```python
from build123d import *

# Parameters (mm, degrees)
SKETCH_R  = 0.7
PAD_DEPTH = 0.25


with BuildPart() as part:
    # Sketch → Pad (new body, symmetric)
    with BuildSketch(Plane.XZ):
        with BuildLine():
            Line((-1.2, 7), (-1.2, 0))
            Line((-1.2, 0), (-0.45, 0))
            Line((-0.45, 0), (-0.45, -2.55))
            ThreePointArc((-0.45, -2.55), (0, -3), (0.45, -2.55))
            Line((0.45, 0), (0.45, -2.55))
            Line((0.45, 0), (1.2, 0))
            Line((1.2, 0), (1.2, 7))
            Line((1.2, 7), (0.7, 7))
            Line((0.7, 7), (0.7, 5.775))
            ThreePointArc((-0.7, 5.775), (0, 5.075), (0.7, 5.775))
            Line((-0.7, 5.775), (-0.7, 7))
            Line((-0.7, 7), (-1.2, 7))
        make_face()
        with Locations((0, 2.3331)):
            Circle(SKETCH_R, mode=Mode.SUBTRACT)
    extrude(amount=PAD_DEPTH, both=True)


solid = part.part
```
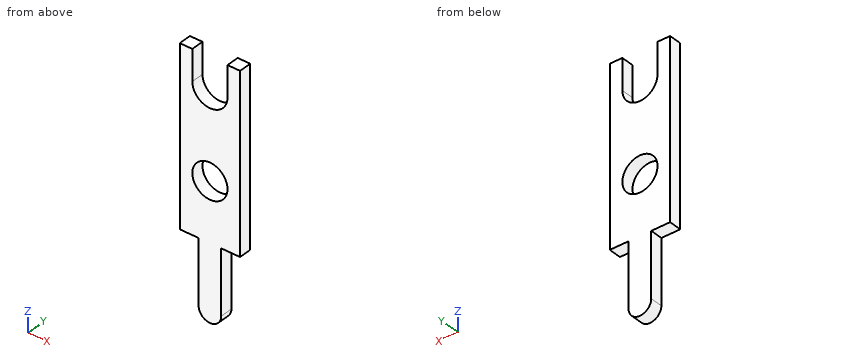
CAD build for the part. Positions are in the model's coordinates, mm. Give positions to 0.01 mm unless a question says otherwise; leave off trailing zeros. Order: outer loops, then holes, each group sorted by start corner. A loop starts at its lowest first (then second) coordinate and runs counter-clockwise, first axis right, second up.
(1) Drill centre lines: L1, parallel to Z at x = 0, y = 0.1 (3 decimals); L2, parallel to X at y = 0.05, z = 5.75; L3, parallel to X at y = 0.1, z = -1.75. Where is each one in solid material? Low to high.
(2) Saw through at B-B, the plane z = 2.75. Give the cut face in (x, y), then the cut area to 3 significant figures.
(3) Saw through at C-C, the plane y = 0.1. Give the cut face in (x, z) (3 decimals).
(4) Saw through at D-D, the plane x = 0.9. Give the cut face in (y, z), then the cut area to 3 significant figures.
(5) Saw through at A-A, the plane x = 0. Give the cut face in (y, z) (3 decimals), then the cut area to 3 significant figures.
Results found:
1. L1: z = -3 to 1.633, 3.033 to 5.075
1. L2: x = -1.2 to -0.7, 0.7 to 1.2
1. L3: x = -0.45 to 0.45
2. outline: (-1.2, -0.25) - (-0.56, -0.25) - (-0.56, 0.25) - (-1.2, 0.25) - close; (0.56, -0.25) - (1.2, -0.25) - (1.2, 0.25) - (0.56, 0.25) - close
2. area: 0.638 mm2
3. outline: (-1.2, 0) - (-0.45, 0) - (-0.45, -2.55) arc R0.45 ccw to (0.45, -2.55) - (0.45, 0) - (1.2, 0) - (1.2, 7) - (0.7, 7) - (0.7, 5.775) arc R0.7 cw to (-0.7, 5.775) - (-0.7, 7) - (-1.2, 7) - close; hole circle Ø1.4 at (0, 2.333)
4. outline: (-0.25, 0) - (0.25, 0) - (0.25, 7) - (-0.25, 7) - close
4. area: 3.50 mm2
5. outline: (-0.25, -3) - (0.25, -3) - (0.25, 1.633) - (-0.25, 1.633) - close; (-0.25, 3.033) - (0.25, 3.033) - (0.25, 5.075) - (-0.25, 5.075) - close
5. area: 3.34 mm2
